The listing builds one solid part. Answer for the finished solid, in the listing's coordinates (mm). Face numbers are marked on the shaded views. A direction names the side the tool comes from. Coordinates: 2 decimals unless noted, no trailing zeros. Order: outer loops, then holes, each group sorted by start corner. A loop starts at its lowest first (then second) coordinate and runs counter-clockwise, first axis right, second up. Notation, with made-up numbers: (82.25, 18) -> (117.25, 18) arc R18 ccw to (117.25, 41) -> close; hole circle Ø11 at (60.5, -12.5). An arc over 180 degrees is marked (long way). Write each question's results on one line, items separated by ' | '. Start each with the question number.
(1) A tool of negligible diameter and unlimited length cuts with its end or side. For the marked faces 1 and 2, from which of +Z, -Z, +X, -X, +Y, -Y can it reach the whole face along a straight path? Write none if from no direction.
(2) The part is cut by section D-D, the plane z = 8.75. Give the vertices of the cut face in (x, y), then the cut area to 3 significant figures.
(3) Straight lines are drawn through the part: L1, parallel to Y at x = 16.5, z = -4.5; L2, parallel to X at y = 1.5, z = -4.25; L3, parallel to Y at x = -31, z = 4.25. For each, find the intervals that lie inside material, in ascending order.
(4) The part is cut by section B-B, the plane z = -5. Give the vertices of the cut face in (x, y), then the cut area to 3 significant figures.
(5) The part is cut by section A-A, the plane x = -5. Give the vertices of the cut face in (y, z), then the cut area to 3 significant figures.
(6) The part is cut by section C-C, the plane x = -13.5. Give the vertices of the cut face in (y, z), then the cut area to 3 significant figures.
(7) Given pin 1 (1 mm diameter, centred on x = -26, z = -4, fed in from +Y); pin 2 (1.2 mm diameter, centred on y = 0, z = -0.5, fed in from +X); pin 3 (1.2 mm diameter, centred on y = 0, z = 0, fed in from -X), each flat-ended and moving along its own axis, determine where each tip first touches the part or whether it passes through.
```python
from build123d import *

# Parameters (mm, degrees)
EXTRUDE_THIN1_DEPTH = 12.7
FILLET1_R           = 8.89
SKETCH2_W           = 25.4
SKETCH2_H           = 2.4384
CUT_EXTRUDE1_DEPTH  = 44.175296885


with BuildPart() as part:
    # Sketch1 → Extrude-Thin1 (new, symmetric)
    with BuildSketch(Plane.XY):
        with BuildLine():
            Line((-40.282118102, -5.54193795), (-33.251527154, -1.482824374))
            ThreePointArc((-33.251527154, -1.482824374), (-31.542374199, -0.774870039), (-29.708227154, -0.5334))
            Line((-29.708227154, -0.5334), (29.708227154, -0.5334))
            ThreePointArc((29.708227154, -0.5334), (31.818482356, -0.255579632), (33.784927154, 0.558948473))
            Line((33.784927154, 0.558948473), (40.815518102, 4.61806205))
            Line((40.815518102, 4.61806205), (40.282118102, 5.54193795))
            Line((40.282118102, 5.54193795), (33.251527154, 1.482824374))
            ThreePointArc((33.251527154, 1.482824374), (31.542374199, 0.774870039), (29.708227154, 0.5334))
            Line((29.708227154, 0.5334), (-29.708227154, 0.5334))
            ThreePointArc((-29.708227154, 0.5334), (-31.818482356, 0.255579632), (-33.784927154, -0.558948473))
            Line((-33.784927154, -0.558948473), (-40.815518102, -4.61806205))
            Line((-40.815518102, -4.61806205), (-40.282118102, -5.54193795))
        make_face()
    extrude(amount=EXTRUDE_THIN1_DEPTH, both=True)

    # Fillet1
    fillet1_edges = [part.edges().sort_by_distance(p)[0] for p in [
        (40.548818102, 5.08, -12.7),
        (40.548818102, 5.08, 12.7),
        (-40.548818102, -5.08, -12.7),
        (-40.548818102, -5.08, 12.7),
    ]]
    fillet(fillet1_edges, radius=FILLET1_R)

    # Sketch2 → Cut-Extrude1 (cut, through all)
    with BuildSketch(Plane(origin=(0, 0.5334, 0), x_dir=(1, 0, 0), z_dir=(0, 1, 0))):
        Rectangle(SKETCH2_W, SKETCH2_H)
    extrude(amount=-CUT_EXTRUDE1_DEPTH, mode=Mode.SUBTRACT)


solid = part.part
```
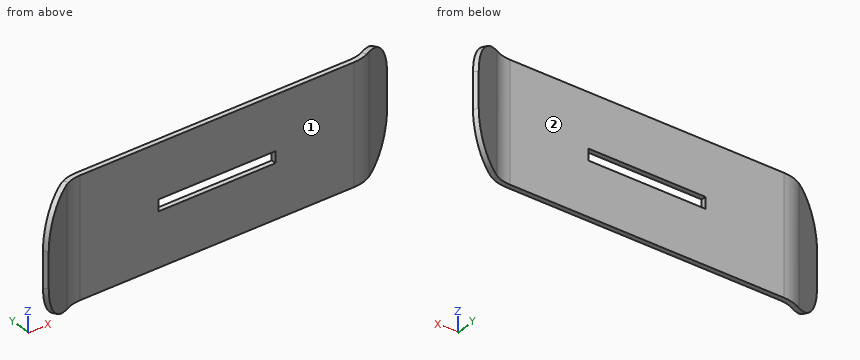
Established:
1) face 1: +Z, -Z, +X, -Y | face 2: +Z, -Z, -X, +Y
2) outline: (-39.52, -3.87) -> (-38.98, -4.79) -> (-33.25, -1.48) arc R7.09 cw to (-29.71, -0.53) -> (29.71, -0.53) arc R8.15 ccw to (33.78, 0.56) -> (39.52, 3.87) -> (38.98, 4.79) -> (33.25, 1.48) arc R7.09 cw to (29.71, 0.53) -> (-29.71, 0.53) arc R8.15 ccw to (-33.78, -0.56) -> close | area: 86.0 mm^2
3) L1: y = -0.53 to 0.53 | L2: x = 33.28 to 35.41 | L3: y = -0.65 to 0.43
4) outline: (-40.75, -4.58) -> (-40.21, -5.5) -> (-33.25, -1.48) arc R7.09 cw to (-29.71, -0.53) -> (29.71, -0.53) arc R8.15 ccw to (33.78, 0.56) -> (40.75, 4.58) -> (40.21, 5.5) -> (33.25, 1.48) arc R7.09 cw to (29.71, 0.53) -> (-29.71, 0.53) arc R8.15 ccw to (-33.78, -0.56) -> close | area: 89.0 mm^2
5) outline: (-0.53, -12.7) -> (0.53, -12.7) -> (0.53, -1.22) -> (-0.53, -1.22) -> close; (-0.53, 1.22) -> (0.53, 1.22) -> (0.53, 12.7) -> (-0.53, 12.7) -> close | area: 24.5 mm^2
6) outline: (-0.53, -12.7) -> (0.53, -12.7) -> (0.53, 12.7) -> (-0.53, 12.7) -> close | area: 27.1 mm^2
7) pin 1: stops at y = 0.53 | pin 2: stops at x = 33.86 | pin 3: stops at x = -33.86
